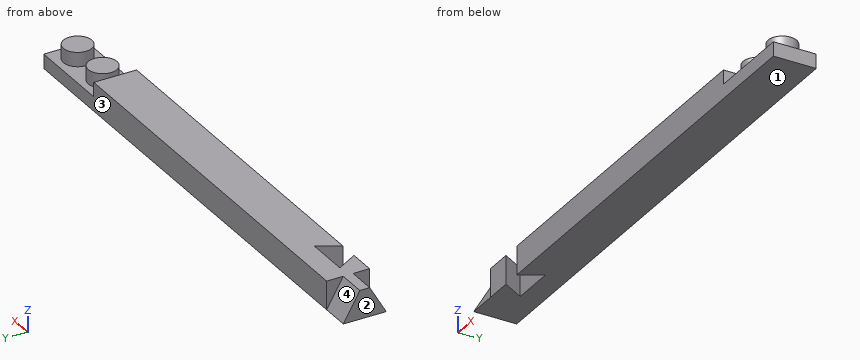
```python
from build123d import *

# Parameters (mm, degrees)
SKETCH_W        = 170
SKETCH_H        = 15
PAD_DEPTH       = 10
SKETCH001_W     = 35
SKETCH001_H     = 25
POCKET_DEPTH    = 5
SKETCH002_R     = 5
PAD001_DEPTH    = 5
PAD002_DEPTH    = 10
POCKET001_DEPTH = 10


with BuildPart() as part:
    # Sketch → Pad (new body)
    with BuildSketch(Plane.XY):
        with Locations((-20.728933, -1.58076)):
            Rectangle(SKETCH_W, SKETCH_H)
    extrude(amount=PAD_DEPTH)

    # Sketch001 (on Face6 of Pad) → Pocket (cut)
    with BuildSketch(Plane.XY.offset(10)):
        with Locations((51.771067, -1.58076)):
            Rectangle(SKETCH001_W, SKETCH001_H)
    extrude(amount=-POCKET_DEPTH, mode=Mode.SUBTRACT)

    # Sketch002 (on Face7 of Pocket) → Pad001 (join)
    with BuildSketch(Plane.XY.offset(5)):
        with Locations((56.771067, -1.58076)):
            Circle(SKETCH002_R)
        with Locations((41.771067, -1.58076)):
            Circle(SKETCH002_R)
    extrude(amount=PAD001_DEPTH)

    # Sketch003 (on Face1 of Pad001) → Pad002 (join)
    with BuildSketch(Plane(origin=(-105.728933, 0, 0), x_dir=(0, -1, 0), z_dir=(-1, 0, 0))):
        Polygon((-5.91924, 0), (-0.145737, 10), (3.307257, 10), (9.08076, 0), align=None)
    extrude(amount=PAD002_DEPTH)

    # Sketch004 (on Face3 of Pad002) → Pocket001 (cut)
    with BuildSketch(Plane.XY.offset(10)):
        Polygon((-93.103933, -14.787648), (-100.728933, -1.58076), (-85.478933, -1.58076), align=None)
    extrude(amount=-POCKET001_DEPTH, mode=Mode.SUBTRACT)


solid = part.part
```
For this review, take the finished solid that the model builds, in its own axes (mm). Face numbers are marked on the shaded views. A direction names the side the tool comes from. Round coordinates to 2 decimals unless told otherwise and drop trailing zeros. Write each loop counter-clockwise with the first axis right and the second up, starting at its lowest first coordinate (ties: lowest second). Pieces come first, ordered by that corner, then holes. Notation, with made-up numbers: M 16,51 L 36,51 A21 cw 36,81 Z; hole C 68.5,80.25 d4. An arc over 180 degrees is marked long. One line per item, written item: value. Start each with the question number.
(1) The part is to be moulded in two halves that separate along X. For the marked faces 1 and 2, say which applies: released by +X, released by -X, zero draft, split by the parting line, or undercut.
(2) Wall thickness on line 1 (X direction, y = -5.25, z = 7.5); line 2 (X direction, y = -2.5, z = 6.75); line 3 (X direction, y = -0.5, z = 6): over which ranges is each line inside the solid? List them lowest first.
(3) Machinability: for the marked faces 3 and 4, which of the approach directions +Z, -Z, +X, -X, +Y, -Y give a long, thin tool a straight path to every point of the face, cutting with its end or side? Answer none if there is none.
(4) We need section A-A (z = 6.5). Give the boundary of the cut face in (x, y), and give its area (3 significant figures).
(5) We need section B-B (x = -93). Give the boundary of the cut face in (y, z), and give its area (3 significant figures).
Result:
1. face 1: zero draft
1. face 2: released by -X
2. line 1: -105.73 to -98.61, -87.6 to 34.27, 38.37 to 45.17, 53.37 to 60.17
2. line 2: -115.73 to -100.2, -86.01 to 34.27, 36.86 to 46.69, 51.86 to 61.69
2. line 3: -115.73 to 34.27, 36.89 to 46.65, 51.89 to 61.65
3. face 3: +Z, -Z, +X, -X, +Y
3. face 4: +Z, -X, +Y
4. outline: M -115.73,-5.33 L -105.73,-5.33 L -105.73,-9.08 L -96.4,-9.08 L -100.73,-1.58 L -85.48,-1.58 L -89.81,-9.08 L 34.27,-9.08 L 34.27,5.92 L -105.73,5.92 L -105.73,2.17 L -115.73,2.17 Z; C 41.77,-1.58 d10; C 56.77,-1.58 d10
4. area: 2,250 mm²
5. outline: M -1.58,0 L 5.92,0 L 5.92,10 L -1.58,10 Z
5. area: 75.0 mm²
